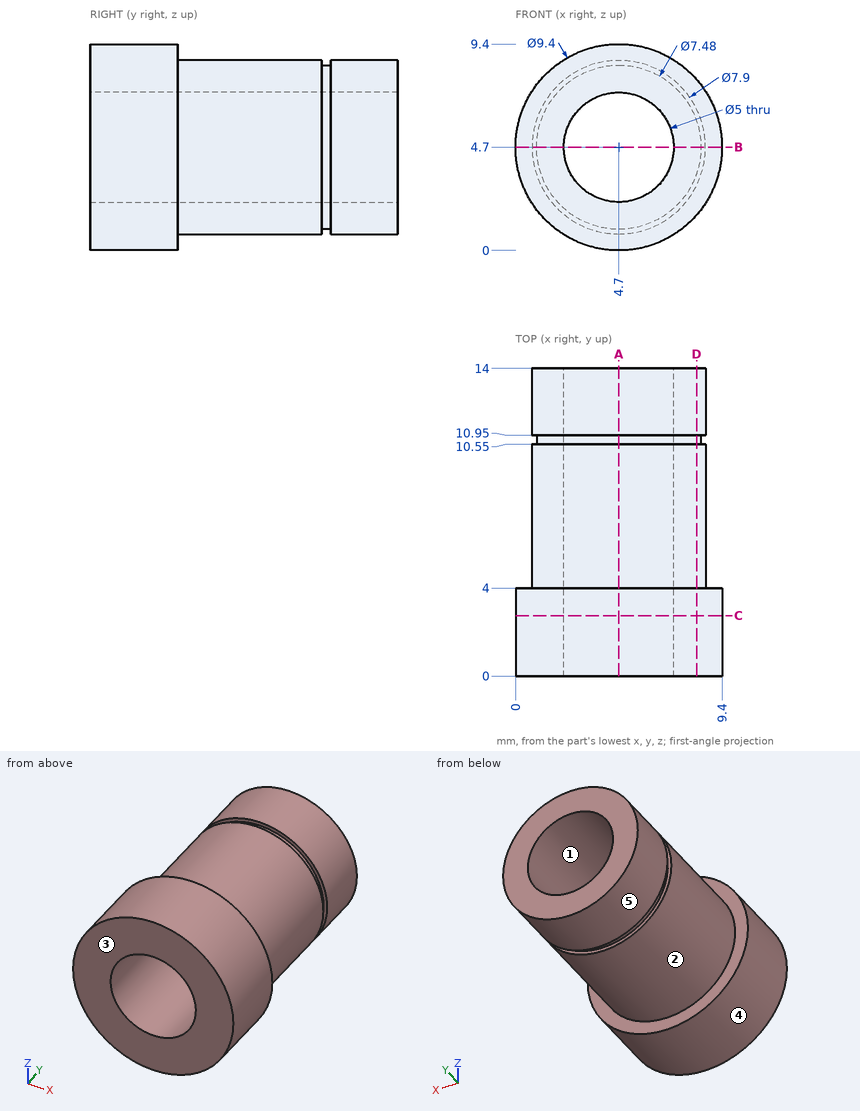
Part print with two shaded views. Sizes in mm from the minimum x, y, z corner. A direction names the side the tool comes from. Give positions to 0.01 mm unless a question says otherwise; leave off trailing zeros. Loops run counter-clockwise (first coordinate to the right, second up) from the corner with the lowest first, then second, coordinate; pieces in that order, holes last. Notation, with made-up numbers: (-18.75, 19.5) - (-13.75, 19.5) arc R12 cw to (-13.75, 42.5) - close; hole circle Ø8 at (21.25, 45). An arc over 180 degrees is marked (long way). Put each result on its own line as item: value.
Q1. Probe line 1 along X through (y, z) = (8.5, 4.7); line 2 along Y through (x, z) = (0.5, 3.5). List the from-to ranges inside material, lowest first.
Filled in:
line 1: x = 0.75 to 2.2, 7.2 to 8.65
line 2: y = 0 to 4
Q2. Slice it at C-C (y = 2.75). Give the cut face in (x, z), plus the area to 3 significant figures.
Filled in:
outline: circle Ø9.4 at (4.7, 4.7); hole circle Ø5 at (4.7, 4.7)
area: 49.8 mm²
Q3. Slice it at D-D (x = 8.25). Give the cut face in (y, z), plus the area to 3 significant figures.
Filled in:
outline: (0, 1.62) - (4, 1.62) - (4, 2.97) - (10.55, 2.97) - (10.55, 3.52) - (10.95, 3.52) - (10.95, 2.97) - (14, 2.97) - (14, 6.43) - (10.95, 6.43) - (10.95, 5.88) - (10.55, 5.88) - (10.55, 6.43) - (4, 6.43) - (4, 7.78) - (0, 7.78) - close
area: 58.8 mm²
Q4. Slice it at A-A (x = 4.7). Give the cut face in (y, z).
Filled in:
outline: (0, 0) - (4, 0) - (4, 0.75) - (10.55, 0.75) - (10.55, 0.96) - (10.95, 0.96) - (10.95, 0.75) - (14, 0.75) - (14, 2.2) - (0, 2.2) - close; (0, 7.2) - (14, 7.2) - (14, 8.65) - (10.95, 8.65) - (10.95, 8.44) - (10.55, 8.44) - (10.55, 8.65) - (4, 8.65) - (4, 9.4) - (0, 9.4) - close
Q5. Tool access for the marked faces 4 and 5: list every direction of +Z, -Z, +X, -X, +Y, -Y with a clear straight run to the whole face (end or side of a thin tool).
Filled in:
face 4: +Y, -Y
face 5: +Y
Q6. Mould opens along X. For the marked faces 1, 2 and 3 say: pulls with the +X half, pulls with the -X half, needs draft (parallel to the pull), parting line crosses it, or undercut.
Filled in:
face 1: undercut
face 2: parting line crosses it
face 3: needs draft
Q7. Flat gauge pins, fed straight in: pin 1 (4.5 mm diameter, centred on x = 4.7, z = 4.7, fed in from +Y); pin 2 (1 mm diameter, centred on y = 9.5, z = 5, fed in from -X); pin 3 (2 mm diameter, centred on x = 3, y = 12.5, fed in from -Z); pin 4 (1 mm diameter, centred on x = 4, y = 3, fed in from -Z). Where does each tip first touch, or does it go through?
Filled in:
pin 1: passes through
pin 2: stops at x = 0.75
pin 3: stops at z = 0.81
pin 4: stops at z = 0
Q8. Slice it at B-B (z = 4.7). Give the cut face in (x, y), plus the area to 3 significant figures.
Filled in:
outline: (0, 0) - (2.2, 0) - (2.2, 14) - (0.75, 14) - (0.75, 10.95) - (0.96, 10.95) - (0.96, 10.55) - (0.75, 10.55) - (0.75, 4) - (0, 4) - close; (7.2, 0) - (9.4, 0) - (9.4, 4) - (8.65, 4) - (8.65, 10.55) - (8.44, 10.55) - (8.44, 10.95) - (8.65, 10.95) - (8.65, 14) - (7.2, 14) - close
area: 46.4 mm²
